Build history of the part. All positions in model axes, mm. Face numbers are marked on the shaded views. A direction names the side the tool comes from. Round coordinates to 2 decimals unless told otherwise and drop trailing zeros. Loops run counter-clockwise (first coordinate to the right, second up) from the corner with the lowest first, then second, coordinate; pieces in that order, holes last.
from build123d import *

# Parameters (mm, degrees)
SKETCH_1_W          = 120
SKETCH_1_H          = 120
EXTRUDE_1_DEPTH     = 5
SKETCH_2_W          = 50
SKETCH_2_H          = 50
EXTRUDE_2_DEPTH     = 245
SKETCH_3_W          = 43
SKETCH_3_H          = 43
CUT_EXTRUDE_2_DEPTH = 250
SKETCH_6_W          = 50
SKETCH_6_H          = 50
SKETCH_6_W_2        = 47
SKETCH_6_H_2        = 47
CUT_EXTRUDE_5_DEPTH = 50
SKETCH_7_W          = 47
SKETCH_7_H          = 47
SKETCH_7_W_2        = 45.5
SKETCH_7_H_2        = 45.5
CUT_EXTRUDE_8_DEPTH = 50


with BuildPart() as part:
    # 草图1 → 凸台-拉伸1 (new body)
    with BuildSketch(Plane.XY):
        Rectangle(SKETCH_1_W, SKETCH_1_H)
    extrude(amount=EXTRUDE_1_DEPTH)

    # 草图2 → 凸台-拉伸2 (add)
    with BuildSketch(Plane.XY.offset(5)):
        Rectangle(SKETCH_2_W, SKETCH_2_H)
    extrude(amount=EXTRUDE_2_DEPTH)

    # 草图3 → 切除-拉伸2 (cut)
    with BuildSketch(Plane.XY.offset(250)):
        Rectangle(SKETCH_3_W, SKETCH_3_H)
    extrude(amount=-CUT_EXTRUDE_2_DEPTH, mode=Mode.SUBTRACT)

    # 草图6 → 切除-拉伸5 (cut)
    with BuildSketch(Plane.XY.offset(250)):
        Rectangle(SKETCH_6_W, SKETCH_6_H)
        Rectangle(SKETCH_6_W_2, SKETCH_6_H_2, mode=Mode.SUBTRACT)
    extrude(amount=-CUT_EXTRUDE_5_DEPTH, mode=Mode.SUBTRACT)

    # 草图7 → 切除-拉伸8 (cut)
    with BuildSketch(Plane.XY.offset(250)):
        Rectangle(SKETCH_7_W, SKETCH_7_H)
        Rectangle(SKETCH_7_W_2, SKETCH_7_H_2, mode=Mode.SUBTRACT)
    extrude(amount=-CUT_EXTRUDE_8_DEPTH, mode=Mode.SUBTRACT)


solid = part.part
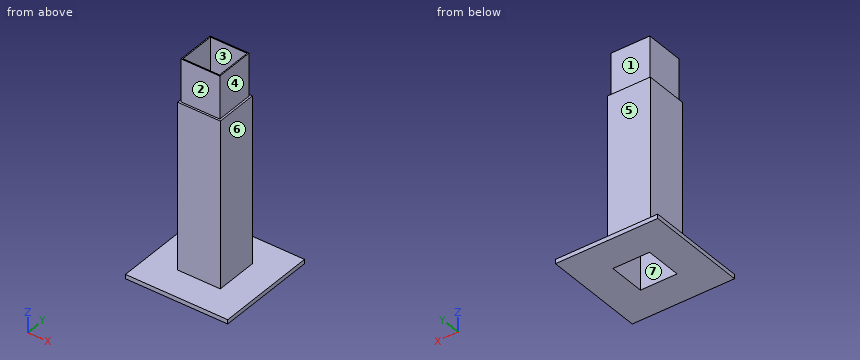
(1) Which spindle directions (+Z, -Z, +X, -X, +Y, -Y) get a long thin tool onto all of the face, cutting with end or side? Do the marked faces 5, 6 and 7. Say none if no direction does.
Responses:
face 5: +Z, +X, -X, +Y
face 6: +Z, +X, +Y, -Y
face 7: +Z, -Z
(2) Probe line 1 (Y direction, x = -4.5, z = 47.5); line 2 (X direction, y = -14, z = 213). List the from-to ranges inside material, lowest first.
Responses:
line 1: y = -25 to -21.5, 21.5 to 25
line 2: x = -22.75 to -21.5, 21.5 to 22.75
(3) Slice it at A-A on y = 8.5. List the corners of the cut face in (x, z), plus the area to 4 significant figures.
Responses:
outline: (-60, 0) - (-21.5, 0) - (-21.5, 250) - (-22.75, 250) - (-22.75, 200) - (-25, 200) - (-25, 5) - (-60, 5) - close; (21.5, 0) - (60, 0) - (60, 5) - (25, 5) - (25, 200) - (22.75, 200) - (22.75, 250) - (21.5, 250) - close
area: 1,875 mm2
(4) Slice it at B-B on z = 36.5. List the corners of the cut face in (x, y), plus the area to 3 significant figures.
Responses:
outline: (-25, -25) - (25, -25) - (25, 25) - (-25, 25) - close; hole (-21.5, -21.5) - (21.5, -21.5) - (21.5, 21.5) - (-21.5, 21.5) - close
area: 651 mm2
(5) Slice it at D-D on x = 41. List the corners of the cut face in (y, z).
Responses:
outline: (-60, 0) - (60, 0) - (60, 5) - (-60, 5) - close
(6) Pin check, flat tips, straight feed: P1, Ø3, axis at x = -8, z = 29.5, coming from the -Y side; P2, Ø21.5, axis at x = 2, z = 159, coming from the +Y side; P3, Ø1.5, axis at x = 26.5, z = 151.5, coming from the -Y side; P4, Ø1, axis at y = -17, z = 201, coming from the -X side. Stop position of each tip, or through.
Responses:
P1: stops at y = -25
P2: stops at y = 25
P3: passes through
P4: stops at x = -22.75
(7) Pull direction Y, two halves, no side cores. Call the marked faces 1, 2, 3 and 4: +Y half, -Y half, draft (parallel to the pull), parting line (faces both ways), or undercut.
Responses:
face 1: +Y half
face 2: -Y half
face 3: undercut
face 4: draft
